Read the model definition and answer for the solid it produces. Units are mm, in the model's axes. A direction names the side the tool comes from. Coordinates: 2 decimals unless noted, no trailing zeros. Loops run counter-clockwise (first coordinate to the right, second up) from the corner with the lowest first, then second, coordinate; pieces in that order, holes last. Notation, with made-up numbers: (-15, 0) - (18, 0) arc R19 ccw to (18, 23) - close; hole circle Ø4 at (34, 10). An arc over 180 degrees is marked (long way). Use CSV: the item, a comma, the result in double quotes.
```python
from build123d import *

# Parameters (mm, degrees)
F1_DEPTH = 3
F2_DEPTH = 1
F3_DEPTH = 6
F0_W     = 15.8
F0_H     = 2
F4_DEPTH = 3.6
F7_DEPTH = 1


with BuildPart() as f1:
    # F0 (on Top) → F1 (new body)
    with BuildSketch(Plane.XY):
        Polygon((48, 20.5), (0, 20.5), (0, 4), (54, 4), (54, 14.5), (48, 14.5), align=None)
    extrude(amount=F1_DEPTH)

    # F0 (on Top) → F2 (join)
    with BuildSketch(Plane.XY):
        Polygon((0, 24.5), (0, 20.5), (48, 20.5), (48, 14.5), (54, 14.5), (54, 4), (0, 4), (0, 0), (48, 0), (48, -2), (38, -2), (38, -7), (40.6, -7), (56.4, -7), (59, -7), (59, -2), (54, -2), (54, 0), (59, 0), (59, 24.5), (54, 24.5), (54, 26.5), (59, 26.5), (59, 31.5), (56.4, 31.5), (40.6, 31.5), (38, 31.5), (38, 26.5), (48, 26.5), (48, 24.5), align=None)
        Polygon((38, 33.5), (40.6, 33.5), (56.4, 33.5), (59, 33.5), (59, 35.3), (56.4, 35.3), (40.6, 35.3), (38, 35.3), align=None)
        Polygon((56.4, -9), (40.6, -9), (38, -9), (38, -10.8), (40.6, -10.8), (56.4, -10.8), (59, -10.8), (59, -9), align=None)
    extrude(amount=F2_DEPTH)

    # F0 (on Top) → F3 (join)
    with BuildSketch(Plane.XY):
        Polygon((0, 4), (0, 20.5), (0, 24.5), (48, 24.5), (48, 26.5), (38, 26.5), (36, 26.5), (-2, 26.5), (-2, -2), (36, -2), (38, -2), (48, -2), (48, 0), (0, 0), align=None)
        Polygon((36, 26.5), (38, 26.5), (38, 31.5), (40.6, 31.5), (40.6, 33.5), (38, 33.5), (38, 35.3), (40.6, 35.3), (40.6, 37.3), (36, 37.3), align=None)
        Polygon((56.4, 33.5), (56.4, 31.5), (59, 31.5), (59, 26.5), (61, 26.5), (61, 37.3), (56.4, 37.3), (56.4, 35.3), (59, 35.3), (59, 33.5), align=None)
        Polygon((61, 26.5), (59, 26.5), (54, 26.5), (54, 24.5), (59, 24.5), (59, 0), (54, 0), (54, -2), (59, -2), (61, -2), align=None)
        Polygon((59, -7), (56.4, -7), (56.4, -9), (59, -9), (59, -10.8), (56.4, -10.8), (56.4, -12.8), (61, -12.8), (61, -2), (59, -2), align=None)
        Polygon((38, -7), (38, -2), (36, -2), (36, -12.8), (40.6, -12.8), (40.6, -10.8), (38, -10.8), (38, -9), (40.6, -9), (40.6, -7), align=None)
    extrude(amount=F3_DEPTH)

    # F0 (on Top) → F4 (join)
    with BuildSketch(Plane.XY):
        with Locations((48.5, 36.3)):
            Rectangle(F0_W, F0_H)
        with Locations((48.5, 32.5)):
            Rectangle(F0_W, F0_H)
        with Locations((48.5, -8)):
            Rectangle(F0_W, F0_H)
        with Locations((48.5, -11.8)):
            Rectangle(F0_W, F0_H)
    extrude(amount=F4_DEPTH)

    # F6 (on face) + F5 (on face) → F7 (join)
    with BuildSketch(Plane.XY.offset(6)):
        Polygon((61, 37.3), (56.4, 37.3), (56.4, 35.3), (59, 35.3), (59, 33.5), (56.4, 33.5), (56.4, 31.5), (61, 31.5), align=None)
        Polygon((61, -7), (56.4, -7), (56.4, -9), (59, -9), (59, -10.8), (56.4, -10.8), (56.4, -12.8), (61, -12.8), align=None)
    with BuildSketch(Plane.XY.offset(6)):
        Polygon((40.6, 37.3), (36, 37.3), (36, 31.5), (38, 31.5), (40.6, 31.5), (40.6, 33.5), (38, 33.5), (38, 35.3), (40.6, 35.3), align=None)
        Polygon((38, -7), (36, -7), (36, -12.8), (40.6, -12.8), (40.6, -10.8), (38, -10.8), (38, -9), (40.6, -9), (40.6, -7), align=None)
    extrude(amount=F7_DEPTH)


solid = f1.part
```
Q1. Find the intervals of material crossed by probe 1 along Y at (x, z) = (25.5, 2.75); probe 2 along X at (y, z) = (35, 4); probe 3 along X at (y, z) = (20, 1.5), in increasing order. Write a range as [from, to].
Reported:
probe 1,"y = [-2, 0], [4, 20.5], [24.5, 26.5]"
probe 2,"x = [36, 38], [59, 61]"
probe 3,"x = [-2, 48], [59, 61]"
Q2. The part is cut by section D-D on y = 17. Determine the outline of the cut face in (x, z).
Reported:
outline,"(-2, 0) - (61, 0) - (61, 6) - (59, 6) - (59, 1) - (48, 1) - (48, 3) - (0, 3) - (0, 6) - (-2, 6) - close"
Q3. The part is cut by section A-A on x = 23. Determine the outline of the cut face in (y, z), and give its area (3 significant figures).
Reported:
outline,"(-2, 0) - (26.5, 0) - (26.5, 6) - (24.5, 6) - (24.5, 1) - (20.5, 1) - (20.5, 3) - (4, 3) - (4, 1) - (0, 1) - (0, 6) - (-2, 6) - close"
area,"81.5 mm²"
Q4. The part is cut by section B-B on y = -1. Determine the outline of the cut face in (x, z), and give its area (3 significant figures).
Reported:
outline,"(-2, 0) - (61, 0) - (61, 6) - (54, 6) - (54, 1) - (48, 1) - (48, 6) - (-2, 6) - close"
area,"348 mm²"
Q5. For a pull along Y with two mould halves and no side action, classify faces 5 (the face through (56, 24.5, 3)), 6 (the face through (40.6, 36, 5)), 7 (the face through (24, 0, 3)) as +Y half, -Y half, draft (parallel to the pull), parting line (faces both ways), or undercut.
Reported:
face 5,"undercut"
face 6,"draft"
face 7,"undercut"
Q6. The part is cut by section C-C on z = 1.75. Give the number of separate pieces and of enclosed holes in the cut face, and give its area (3 significant figures).
Reported:
separate pieces,"1"
enclosed holes,"3"
area,"1,440 mm²"
Q7. Given P1, Ø2, axis at y = 36.5, z = 5, coming from the -X side; P2, Ø6, axis at x = 15.5, y = 5, coming from the -Z side; P3, Ø5, axis at x = 27, y = 18.5, coming from the +Z side; P4, Ø12, axis at x = 22.5, y = 20.5, coming from the +Z side, each flat-ended and moving along its own axis, determine where each tip first touches the part or whether it passes through.
Reported:
P1,"stops at x = 36"
P2,"stops at z = 0"
P3,"stops at z = 3"
P4,"stops at z = 6"
Q8. A tool of negligible diameter and unlimited length cuts with its end or side. For faces 1 (the face through (48, 31.5, 3)), 2 (the face through (56.4, -12, 5)), 3 (the face through (36, 13, 0)), 4 (the face through (48, 33, 3.6)), from which of +Z, -Z, +X, -X, +Y, -Y can it reach the whole face along a straight path? Write none if from no direction.
Reported:
face 1,"+Z"
face 2,"+Z, -Y"
face 3,"-Z, +X, -X, +Y, -Y"
face 4,"+Z, +Y"
